Geometry: final body of the model. Coordinates: model frame, mm. Round coordinates to 2 decimals unless told otherwise and drop trailing zeros. Write each loop counter-clockwise with the first axis right and the second up, starting at its lowest first coordinate (ties: lowest second). Pieces come first, ordered by that corner, then holes. Notation, with made-up numbers: M 56,13 L 112,13 A20 ccw 112,50 Z; hole C 32,21.5 d6. An arc over 180 degrees is marked long. Use one line per item in the form item = value. Start each with the question number.
Item 1: Section query C-C (z = 1.1). State how many separate pieces and enclosed holes the cut face has, and give its area (3 significant figures).
Item 2: Ray query, probe 1 along Y at (x, z) = (-264.3, 1.75); probe 2 along X at (y, z) = (-18, 2.95); probe 3 along Y at (x, z) = (73, 2.8). Return the intervals inside material, ascending.
Item 3: Section query B-B (y = -73.5). Return loops of the section in (x, z) (1 decimal).
Item 4: Pin query (flat end, axial travel): pin 1 Ø6.5 at (x, y) = (-264.3, 19.25) entering from -Z. Return the tip coordinate at first contact, or that it passes through.
Item 5: Section query A-A (x = 88). Return loops of the section in (y, z) (1 decimal).
Autodesk Inventor part; units mm, degrees
ref_plane "YZ Plane" through (0, 0, 0) normal (1, 0, 0) x (0, 1, 0)
ref_plane "XZ Plane" through (0, 0, 0) normal (0, 1, 0) x (-1, 0, 0)
ref_plane "XY Plane" through (0, 0, 0) normal (0, 0, 1) x (1, 0, 0)
ref_plane "Work Plane1" through (0, 0, 0) normal (0, 0, 1) x (1, 0, 0)
sketch "Sketch1" plane through (0, 0, 0) normal (0, 0, 1) x (1, 0, 0)
  arc A0 (-261.52, -25.4) -> (-260.25, -24.13) centre (-261.52, -24.13) ccw
  line L0 (-261.52, -25.4) -> (-265.66, -25.4)
  arc A1 (-266.93, -24.13) -> (-265.66, -25.4) centre (-265.66, -24.13) ccw
  line L1 (-266.93, -24.13) -> (-266.93, -21.59)
  arc A2 (-265.66, -20.32) -> (-266.93, -21.59) centre (-265.66, -21.59) ccw
  line L2 (-265.66, -20.32) -> (-261.52, -20.32)
  arc A3 (-260.25, -21.59) -> (-261.52, -20.32) centre (-261.52, -21.59) ccw
  line L3 (-260.25, -21.59) -> (-260.25, -24.13)
  circle A4 centre (-264.3, 19.25) radius 3.6
  arc A5 (291.2125, 168.0875) -> (288.0375, 171.2625) centre (288.0375, 168.0875) ccw
  line L4 (288.0375, 171.2625) -> (-288.0375, 171.2625)
  arc A6 (-288.0375, 171.2625) -> (-291.2125, 168.0875) centre (-288.0375, 168.0875) ccw
  line L5 (-291.2125, 168.0875) -> (-291.2125, -168.0875)
  arc A7 (-291.2125, -168.0875) -> (-288.0375, -171.2625) centre (-288.0375, -168.0875) ccw
  line L6 (-288.0375, -171.2625) -> (288.0375, -171.2625)
  arc A8 (288.0375, -171.2625) -> (291.2125, -168.0875) centre (288.0375, -168.0875) ccw
  line L7 (291.2125, -168.0875) -> (291.2125, 168.0875)
  point P0 (0, 0)
extrude "Extrusion1" add sketch "Sketch1" along normal blind 3.175
sketch "Sketch2" plane through (0, 0, 0) normal (0, 0, 1) x (1, 0, 0)
  arc A0 (267.27, -148.59) -> (268.54, -147.32) centre (267.27, -147.32) ccw
  line L0 (268.54, 140.97) -> (268.54, -147.32)
  line L1 (-244.54, 140.97) -> (268.54, 140.97)
  line L2 (-244.54, -147.32) -> (-244.54, 140.97)
  arc A1 (-244.54, -147.32) -> (-243.27, -148.59) centre (-243.27, -147.32) ccw
  line L3 (267.27, -148.59) -> (-243.27, -148.59)
  arc A2 (267.27, -148.59) -> (268.54, -147.32) centre (267.27, -147.32) ccw
  line L4 (268.54, 140.97) -> (268.54, -147.32)
  line L5 (-244.54, 140.97) -> (268.54, 140.97)
  line L6 (-244.54, -147.32) -> (-244.54, 140.97)
  arc A3 (-244.54, -147.32) -> (-243.27, -148.59) centre (-243.27, -147.32) ccw
  line L7 (267.27, -148.59) -> (-243.27, -148.59)
  point P0 (0, 0)
extrude "Extrusion2" cut sketch "Sketch2" along normal blind 3.175
properties material "Wood (Birch)"
Working result:
q1.separate_pieces = 1
q1.enclosed_holes = 3
q1.area = 50,800 mm²
q2.probe_1 = -171.26 to -25.4, -20.32 to 15.65, 22.85 to 171.26
q2.probe_2 = -291.21 to -244.54, 268.54 to 291.21
q2.probe_3 = -171.26 to -148.59, 140.97 to 171.26
q3.outline = M -291.2,0 L -244.5,0 L -244.5,3.2 L -291.2,3.2 Z; M 268.5,0 L 291.2,0 L 291.2,3.2 L 268.5,3.2 Z
q4.pin_1 = through
q5.outline = M -171.3,0 L -148.6,0 L -148.6,3.2 L -171.3,3.2 Z; M 141,0 L 171.3,0 L 171.3,3.2 L 141,3.2 Z
